```python
from build123d import *

# Parameters (mm, degrees)
SKETCH1_W               = 11.5
SKETCH1_H               = 10
SKETCH1_R               = 3.95
BOSS_EXTRUDE1_DEPTH     = 10
SKETCH2_W               = 11.5
SKETCH2_H               = 10
BOSS_EXTRUDE2_DEPTH     = 12
CUT_EXTRUDE1_DEPTH      = 4.25
CUT_EXTRUDE1_DEPTH_BACK = 4.25
SKETCH4_R               = 1.245
CUT_EXTRUDE2_DEPTH      = 18.356554958
CUT_EXTRUDE3_DEPTH      = 17.645194536


with BuildPart() as part:
    # Sketch1 → Boss-Extrude1 (new body)
    with BuildSketch(Plane.XY):
        Rectangle(SKETCH1_W, SKETCH1_H)
        Circle(SKETCH1_R, mode=Mode.SUBTRACT)
    extrude(amount=BOSS_EXTRUDE1_DEPTH)

    # Sketch2 → Boss-Extrude2 (add)
    with BuildSketch(Plane(origin=(0, 0, 0), x_dir=(-1, 0, 0), z_dir=(0, 0, -1))):
        Rectangle(SKETCH2_W, SKETCH2_H)
    extrude(amount=BOSS_EXTRUDE2_DEPTH)

    # Sketch3 → Cut-Extrude1 (cut, two sides: drawn at the far end of the back side and taken through both)
    with BuildSketch(Plane.ZY.offset(-CUT_EXTRUDE1_DEPTH_BACK)):
        with BuildLine():
            Line((-12, -5), (-3.5, -5))
            Line((-3.5, -5), (-3.5, 1.707151991))
            ThreePointArc((-3.5, 1.707151991), (-4.392121597, 3.756542144), (-6.5, 4.5))
            Line((-6.5, 4.5), (-6.5, 5))
            Line((-6.5, 5), (-12, 5))
            Line((-12, 5), (-12, -5))
        make_face()
    extrude(amount=CUT_EXTRUDE1_DEPTH + CUT_EXTRUDE1_DEPTH_BACK, mode=Mode.SUBTRACT)

    # Sketch4 → Cut-Extrude2 (cut, through all)
    with BuildSketch(Plane.ZY.offset(5.75)):
        with Locations((4, 0)):
            Circle(SKETCH4_R)
    extrude(amount=-CUT_EXTRUDE2_DEPTH, mode=Mode.SUBTRACT)

    # Sketch5 → Cut-Extrude3 (cut, through all)
    with BuildSketch(Plane(origin=(0, 5, 0), x_dir=(1, 0, 0), z_dir=(0, 1, 0))):
        with BuildLine():
            ThreePointArc((-2.633913438, 6.5), (-1.408678459, 5.758412878), (0, 5.5))
            Line((0, 5.5), (0, 6.5))
            Line((0, 6.5), (-2.633913438, 6.5))
        make_face()
        with BuildLine():
            Line((0, 6.5), (0, 5.5))
            ThreePointArc((0, 5.5), (1.408678459, 5.758412878), (2.633913438, 6.5))
            Line((2.633913438, 6.5), (0, 6.5))
        make_face()
        with BuildLine():
            Line((-2.633913438, 6.5), (0, 6.5))
            Line((0, 6.5), (2.633913438, 6.5))
            ThreePointArc((2.633913438, 6.5), (3.61969063, 7.841231551), (3.96875, 9.46875))
            ThreePointArc((3.96875, 9.46875), (-1.627518449, 13.08844063), (-2.633913438, 6.5))
        make_face()
    extrude(amount=-CUT_EXTRUDE3_DEPTH, mode=Mode.SUBTRACT)


solid = part.part
```
Here's how the part is built. I have some questions about the finished solid (model axes, mm). A direction names the side the tool comes from. Coordinates: 2 decimals unless noted, no trailing zeros. Order: outer loops, then holes, each group sorted by start corner. A loop starts at its lowest first (then second) coordinate and runs counter-clockwise, first axis right, second up. Notation, with made-up numbers: M -13.5,43 L 40.5,43 A16 ccw 40.5,58 Z; hole C -13.5,82 d4. An arc over 180 degrees is marked long. Answer as a JSON object with one key per item and string values. Group by question number.
(1) Which directions (+Z, -Z, +X, -X, +Y, -Y) give clear straight access to the entire face, cutting with the end or side of a thin tool? Please do faces 1 (the face through (0, 0, 0)), 2 (the face through (-4.25, 0, -8)), 3 (the face through (-4, -1, 10)).
(2) Suppose I cut it at C-C, the plane y = 0. Please give me the cut outline in (x, z) (3 decimals), then the cut area to 3 significant figures.
(3) Suppose I cut it at A-A, the plane z = 4. Please give me the cut outline in (x, y) (3 decimals), then the cut area to 3 significant figures.
(4) If we mould it in two halves opening along Y, with no side actions, what happens to faces 4 (the face through (4.74, -0.48, 5.15)), 5 (the face through (0, 5, 2)), 6 (the face through (3.65, -1.51, 4.93)), 7 (the face through (4.25, 0, -8))? For each: released by +Y, released by -Y, zero draft, split by the parting line, or undercut.
(5) For pin 1 (5.5 mm diameter, centred on x = 0, y = -1.5, fed in from -Z); pin 2 (4.5 mm diameter, centred on x = 0, y = 0, fed in from +Z); pin 3 (0.6 mm diameter, centred on x = 3.5, y = 4.5, fed in from -Z), each with a flat end and sliding along its axis, tell me the tip position at first contact or that it passes through.
(6) I need wall thicknesses on probe 1 along X at (y, z) = (0, 6.25); probe 2 along X at (y, z) = (4, -4.75); probe 3 along Z at (x, y) = (4.3, 0) (3 decimals). Which ranges of each line are inside material? Lowest first, please.
(7) Suppose I cut it at B-B, the plane x = 5.25. Please give me the cut outline in (y, z) (3 decimals).
(8) Suppose I cut it at D-D, the plane z = -9. Please give me the cut outline in (x, y), then the cut area to 3 significant figures.
Values found:
{
 "1": {"face 1": "+Z", "face 2": "-Z, -Y", "face 3": "+Z, +X, -X, +Y, -Y"},
 "2": {"outline": "M -5.75,-12 L -4.25,-12 L -4.25,-3.5 L 4.25,-3.5 L 4.25,-12 L 5.75,-12 L 5.75,2.755 L 3.95,2.755 L 3.95,0 L -3.95,0 L -3.95,2.755 L -5.75,2.755 Z; M -5.75,5.245 L -3.95,5.245 L -3.95,10 L -5.75,10 Z; M 3.95,5.245 L 5.75,5.245 L 5.75,10 L 3.95,10 Z", "area": "92.8 mm^2"},
 "3": {"outline": "M -5.75,-5 L 5.75,-5 L 5.75,-1.245 L 3.749,-1.245 A3.95 cw -3.749,-1.245 L -5.75,-1.245 Z; M -5.75,1.245 L -3.749,1.245 A3.95 cw 3.749,1.245 L 5.75,1.245 L 5.75,5 L -5.75,5 Z", "area": "56.7 mm^2"},
 "4": {"face 4": "undercut", "face 5": "released by +Y", "face 6": "undercut", "face 7": "zero draft"},
 "5": {"pin 1": "stops at z = -3.5", "pin 2": "stops at z = 0", "pin 3": "stops at z = -6.5"},
 "6": {"probe 1": "x = -5.75 to -3.95, 3.95 to 5.75", "probe 2": "x = -5.75 to -4.25, 4.25 to 5.75", "probe 3": "z = -12 to 2.755, 5.245 to 10"},
 "7": {"outline": "M -5,-12 L 5,-12 L 5,10 L -5,10 Z; hole C 0,4 d2.49"},
 "8": {"outline": "M -5.75,-5 L -4.25,-5 L -4.25,5 L -5.75,5 Z; M 4.25,-5 L 5.75,-5 L 5.75,5 L 4.25,5 Z", "area": "30.0 mm^2"}
}
